Job drawing, mm, ordinate dimensions from the low corner. One solid piece. A direction names the side the tool comes from. Give positions to 0.01 mm unless a question says otherwise; leave off trailing zeros. Write each loop counter-clockwise with the first axis right and the second up, starting at its lowest first coordinate (ties: lowest second). Pieces come first, ordered by that corner, then holes. Notation, with made-up numbers: (14, -21.5) - (41, -21.5) arc R16 ccw to (41, -1.5) - close; hole circle Ø4 at (84, 77). An arc over 180 degrees is marked (long way). Put each result on its own line as item: value. Start each with the question number.
1. Cut at B-B on x = 9. List the corners of the cut face in (y, z), and give its area (3 significant figures).
2. Mould opens along Z. For the marked faces 1, 2 and 3 say: +Z half, -Z half, draft (parallel to the pull), parting line (faces both ways), or undercut.
3. Cut at D-D on z = 10.5. List the corners of the cut face in (x, y).
4. Wall check: line 1 (Y direction, x = 9, z = 5.5); line 2 (Z direction, x = 16.75, y = 5.5); line 3 (X direction, y = 2.5, z = 13.5). Give the ranges that are in metal, low to high.
5. Drop flat-ended pins along their axis: pin 1 (10 mm diameter, centred on x = 7.5, z = 13.5, fed in from +Y); pin 2 (4.5 mm diameter, centred on x = 9, y = 9, fed in from +Z); pin 3 (3 mm diameter, centred on y = 8.5, z = 4, fed in from +X); pin 4 (5 mm diameter, centred on y = 5.5, z = 12.5, fed in from +X). Give the stop position or say it passes through.
6. Cut at A-A on y = 2. List the corners of the cut face in (x, z).
7. Tool access for the marked faces 4 and 5: list every direction of +Z, -Z, +X, -X, +Y, -Y with a clear straight run to the whole face (end or side of a thin tool).
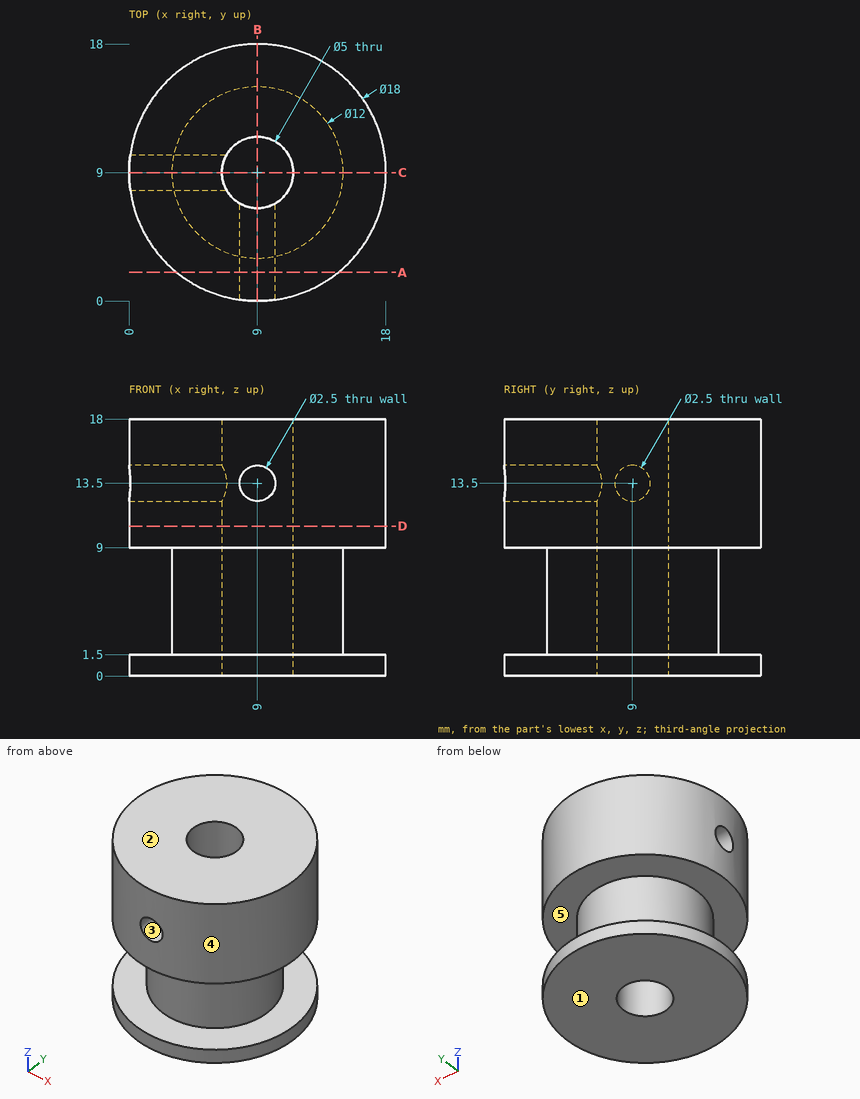
Report:
1. outline: (0, 0) - (6.5, 0) - (6.5, 12.25) - (0, 12.25) - (0, 9) - (3, 9) - (3, 1.5) - (0, 1.5) - close; (0, 14.75) - (6.5, 14.75) - (6.5, 18) - (0, 18) - close; (11.5, 0) - (18, 0) - (18, 1.5) - (15, 1.5) - (15, 9) - (18, 9) - (18, 18) - (11.5, 18) - close
1. area: 173 mm²
2. face 1: -Z half
2. face 2: +Z half
2. face 3: undercut
3. outline: circle Ø18 at (9, 9); hole circle Ø5 at (9, 9)
4. line 1: y = 3 to 6.5, 11.5 to 15
4. line 2: z = 0 to 1.5, 9 to 18
4. line 3: x = 2.78 to 7.75, 10.25 to 15.22
5. pin 1: stops at y = 18
5. pin 2: passes through
5. pin 3: stops at x = 15
5. pin 4: stops at x = 17.94
6. outline: (3.34, 0) - (14.66, 0) - (14.66, 1.5) - (3.34, 1.5) - close; (3.34, 9) - (14.66, 9) - (14.66, 18) - (3.34, 18) - close; hole circle Ø2.5 at (9, 13.5)
7. face 4: +Z, -Z
7. face 5: none
